```python
from build123d import *

# Parameters (mm, degrees)
F0_W     = 50
F0_H     = 60
F1_DEPTH = 40
F3_START = -50
F2_R     = 5
F3_DEPTH = 260


with BuildPart() as f1:
    # F0 (on Top) → F1 (new body)
    with BuildSketch(Plane.XY):
        with Locations((-125, -30)):
            Rectangle(F0_W, F0_H)
    extrude(amount=F1_DEPTH)



with BuildPart() as f1b:
    # F0 (on Top) → F1, piece 2 (new body)
    with BuildSketch(Plane.XY):
        with Locations((185, -30)):
            Rectangle(F0_W, F0_H)
    extrude(amount=F1_DEPTH)


with BuildPart() as f1_1:
    add(f1.part)

    add(f1b.part)  # F3 merges F1b
    # F2 (on face) → F3 (join)
    with BuildSketch(Plane.YZ.offset(210).offset(F3_START)):
        with Locations((-15, 20)):
            Circle(F2_R)
    extrude(amount=-F3_DEPTH)


solid = f1_1.part
```
Here's how the part is built. I have some questions about the finished solid (model axes, mm). A direction names the side the tool comes from. Coordinates: 2 decimals unless noted, no trailing zeros. Loops run counter-clockwise (first coordinate to the right, second up) from the corner with the lowest first, then second, coordinate; pieces in that order, holes last. Notation, with made-up numbers: (24.25, -29.75) - (72.25, -29.75) arc R26 cw to (72.25, -0.75) - close; hole circle Ø6 at (22.25, -1.75). An arc over 180 degrees is marked (long way). Answer as CSV lines item,"result".
Q1. We'd pull the mould along X, two halves only. Please class faces 3 (the face through (160, -30, 20)), 4 (the face through (-150, -30, 20)), 5 (the face through (-125, -60, 20)): pulls with the +X half, pulls with the -X half, needs draft (parallel to the pull), parting line crosses it, or undercut.
Response:
face 3,"undercut"
face 4,"pulls with the -X half"
face 5,"needs draft"
Q2. If I drill on L1, parallel to X at y = -38.5, z = 3; L2, parallel to Z at x = 6.5, y = -12; L3, parallel to Z at x = -68.5, y = -17, over which ranges is the centre line in solid material (lowest first)? Write a range as [from, to].
Response:
L1,"[-150, -100], [160, 210]"
L2,"[16, 24]"
L3,"[15.42, 24.58]"
Q3. If we section it at C-C, the plane z = 20: Write out the boundary of the cut face in (x, y).
Response:
outline,"(-150, -60) - (-100, -60) - (-100, -20) - (160, -20) - (160, -60) - (210, -60) - (210, 0) - (160, 0) - (160, -10) - (-100, -10) - (-100, 0) - (-150, 0) - close"
Q4. For pin 1 (8 mm diameter, centred on x = 73, z = 19, fed in from -Y); pin 2 (5 mm diameter, centred on x = -86.5, z = 21.5, fed in from +Y); pin 3 (1.5 mm diameter, centred on x = 149, z = 16.5, fed in from +Y), each with a flat end and sliding along its axis, tell me the tip position at first contact or that it passes through.
Response:
pin 1,"y = -20"
pin 2,"y = -10"
pin 3,"y = -10.82"
Q5. If we section it at B-B, the plane z = 33: Write out the boundary of the cut face in (x, y).
Response:
outline,"(-150, -60) - (-100, -60) - (-100, 0) - (-150, 0) - close; (160, -60) - (210, -60) - (210, 0) - (160, 0) - close"
Q6. If we section it at A-A, the plane y = -46.5: Write out the boundary of the cut face in (x, z), and give its area (3 significant figures).
Response:
outline,"(-150, 0) - (-100, 0) - (-100, 40) - (-150, 40) - close; (160, 0) - (210, 0) - (210, 40) - (160, 40) - close"
area,"4,000 mm2"
Q7. For faces 1 (the face through (31.82, -16.08, 15.12)), 2 (the face through (-125, -30, 40)), which set-ups out of +Z, -Z, +X, -X, +Y, -Y let a thin tool reach every point of the face, with its end or its side?
Response:
face 1,"none"
face 2,"+Z, +X, -X, +Y, -Y"
Q8. If we section it at D-D, the plane y = -15: Write out the boundary of the cut face in (x, z), and give its area (3 significant figures).
Response:
outline,"(-150, 0) - (-100, 0) - (-100, 15) - (160, 15) - (160, 0) - (210, 0) - (210, 40) - (160, 40) - (160, 25) - (-100, 25) - (-100, 40) - (-150, 40) - close"
area,"6,600 mm2"
